Geometry check sheet. Reference: drawing and pictorial views, mm from the part's lowest x, y, z. A direction names the side the tool comes from. Give positions to 0.01 mm unless a question says otherwise; leave off trailing zeros. Write each loop counter-clockwise with the first axis right and the second up, starting at its lowest first coordinate (ties: lowest second). Pieces come first, ordered by that corner, then holes. Notation, with made-up numbers: (20, -37.5) -> (60, -37.5) arc R30 ccw to (60, -5.5) -> close; hole circle Ø10 at (-29, -39.5). An arc over 180 degrees is marked (long way). Use a Markdown table: item, result. Add a question column.
1. Set-up check for the marked faces 4, 5 and 6: record each of +Z, -Z, +X, -X, +Y, -Y from which the full face is reachable in a straight line by a thin tool's end or side.
2. Cross-section at B-B (z = 50). Enter the section's corners in (x, y).
3. Cross-section at D-D (y = 21.5). Enter the section's corners in (x, z), then the cut area to 3 significant figures.
4. Release check for a two-part mould opening along Y. For the marked faces 1, 2 and 3 record: released by +Y, released by -Y, zero draft, split by the parting line, or undercut.
5. Scan lines: probe 1 along Y at (x, z) = (16, 50); probe 2 along Z at (x, y) = (11, 50); probe 3 along Y at (x, z) = (25.5, 50). Record each from-to range of solid material in increasing order. Write a range as [from, to].
6. Cross-section at A-A (x = 4). Enter the section's corners in (y, z).
7. Gauge pin test, flat ends, axial feed: P1, Ø12, axis at x = 7, z = 49, coming from the -Y side; P2, Ø3.5, axis at y = 50.5, z = 22.5, coming from the -X side; P3, Ø8, axis at x = 6, z = 79, coming from the -Y side. Record the tip position at first contact, or that the pin passes through.
8. Cross-section at C-C (x = 27.5). Enter the section's corners in (y, z).
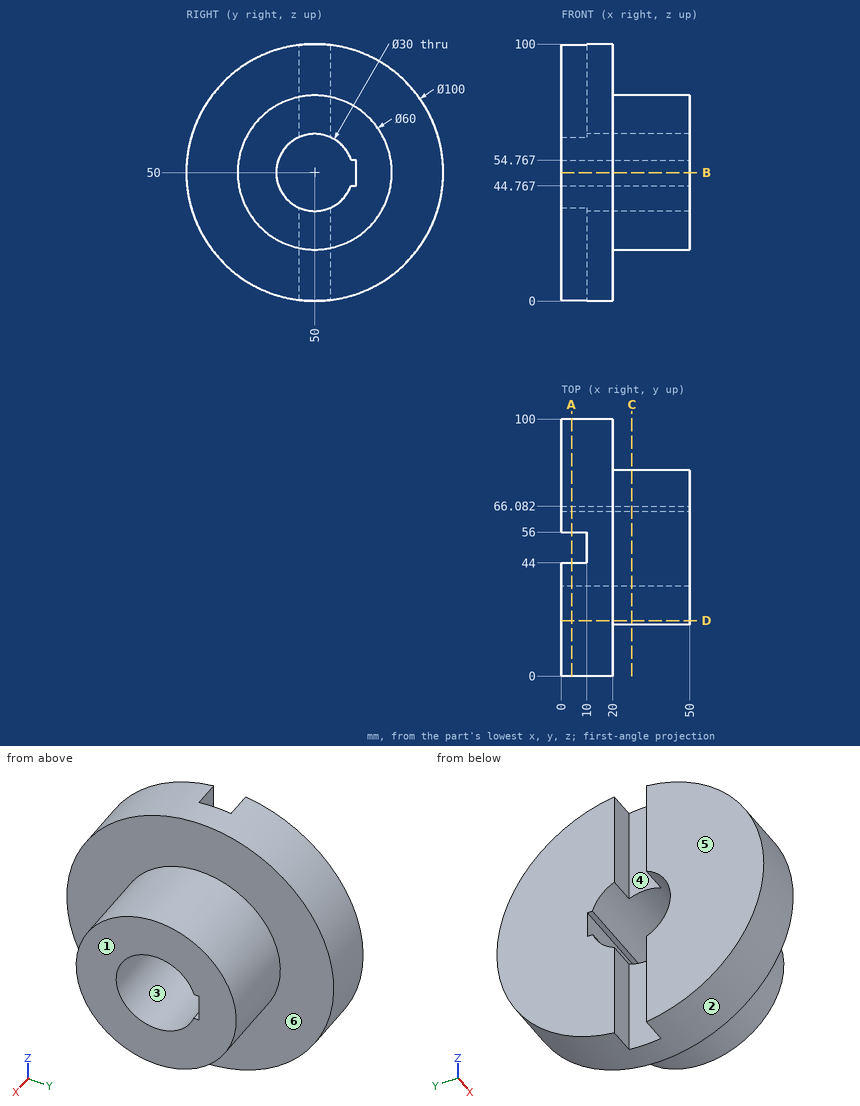
Worked answers:
| question | item | result |
|---|---|---|
| 1 | face 4 | +Z, -Z, -X |
| 1 | face 5 | +Z, -Z, -X, +Y, -Y |
| 1 | face 6 | +X |
| 2 | outline | (0, 0) -> (20, 0) -> (20, 20) -> (50, 20) -> (50, 35) -> (0, 35) -> close; (0, 66.08) -> (50, 66.08) -> (50, 80) -> (20, 80) -> (20, 100) -> (0, 100) -> close |
| 3 | outline | (0, 8.92) -> (20, 8.92) -> (20, 40.63) -> (50, 40.63) -> (50, 59.37) -> (20, 59.37) -> (20, 91.08) -> (0, 91.08) -> close |
| 3 | area | 2,210 mm² |
| 4 | face 1 | zero draft |
| 4 | face 2 | split by the parting line |
| 4 | face 3 | undercut |
| 5 | probe 1 | y = [0, 35], [66.08, 100] |
| 5 | probe 2 | z = [0, 35], [65, 100] |
| 5 | probe 3 | y = [20, 35], [66.08, 80] |
| 6 | outline | (44, 0.36) -> (44, 36.25) arc R15 cw to (44, 63.75) -> (44, 99.64) arc R50 ccw to start; (56, 0.36) arc R50 ccw to (56, 99.64) -> (56, 63.75) arc R15 cw to (64.22, 54.77) -> (66.08, 54.77) -> (66.08, 44.77) -> (64.06, 44.77) arc R15 cw to (56, 36.25) -> close |
| 7 | P1 | stops at y = 0 |
| 7 | P2 | stops at x = 10 |
| 7 | P3 | stops at y = 6.7 |
| 8 | outline | circle Ø60 at (50, 50); hole (64.06, 44.77) -> (66.08, 44.77) -> (66.08, 54.77) -> (64.22, 54.77) arc R15 ccw (long way) to start |
